The listing builds one solid part. Answer for the finished solid, in the listing's coordinates (mm). A direction names the side the tool comes from. Give positions to 0.01 mm unless a question says otherwise; leave off trailing zeros. Order: outer loops, then holes, each group sorted by start corner. A loop starts at its lowest first (then second) coordinate and runs counter-clockwise, first axis right, second up. Notation, with made-up numbers: (-9.75, 9.25) - (6.25, 9.25) arc R23 ccw to (6.25, 44.25) - close; hole circle Ø3 at (38, 17). An arc over 180 degrees is marked (long way). Write each question's results on one line, items separated by ' | '. Start each with the question number.
1. Section C-C (x = -5) is taken. Give the vertices of the cut face in (y, z), and give its area (3 significant figures).
2. Flat-ended cylindrical pins translate along their axes: pin 1 (2.5 mm diameter, centred on y = 26, z = 1.5, fed in from -X); pin 2 (1.5 mm diameter, centred on x = 1, z = 2.5, fed in from +Y); pin 3 (1.5 mm diameter, centred on y = -4.5, z = 3.5, fed in from -X). Find the tip coordinate at first contact, or state that the pin passes through.
3. Which of the six approach directions +Z, -Z, +X, -X, +Y, -Y give full straight-line access (tool end or side, diameter ignored) to faces 1 (the face through (21, 27.5, 2)), 2 (the face through (23, 7, 0))?
4. Section A-A (y = 24) is taken. Give the vertices of the cut face in (x, z), and give its area (3 significant figures).
5. Section B-B (z = 3.05) is taken. State how many separate pieces and enclosed holes the cut face has, and give its area (3 significant figures).
6. Section D-D (x = 17) is taken. Give the vertices of the cut face in (y, z), and give its area (3 significant figures).
7. Determine the mould class of faces 3 (the face through (12.86, 31.93, 2.46)), 4 (the face through (25.76, 25, 2)), 5 (the face through (44.655, 5.676, 2.465)) for opening direction X: released by +X, released by -X, zero draft, split by the parting line, or undercut.
8. Find the intervals of material crossed by L1, parallel to Y at x = 17.5, z = 4.5; L2, parallel to Y at x = 31.5, z = 4; L3, parallel to Y at x = -5, z = 2.45, in increasing order.
from build123d import *

# Parameters (mm, degrees)
SKETCH1_R           = 2
SKETCH1_W           = 10
SKETCH1_H           = 5
BOSS_EXTRUDE1_DEPTH = 5


with BuildPart() as part:
    # Sketch1 → Boss-Extrude1 (new body)
    with BuildSketch(Plane.XY):
        with BuildLine():
            Line((-1.742019887, -10.039309555), (26.411625907, -10.039309555))
            ThreePointArc((26.411625907, -10.039309555), (30.462414048, -9.182127251), (33.818749407, -6.757532642))
            Line((33.818749407, -6.757532642), (43.703561538, 4.140888457))
            ThreePointArc((43.703561538, 4.140888457), (44.664643865, 5.699695686), (44.999999787, 7.5))
            Line((44.999999787, 7.5), (44.999999787, 30.5))
            ThreePointArc((44.999999787, 30.5), (44.41421335, 31.914213562), (42.999999787, 32.5))
            Line((42.999999787, 32.5), (14.260362516, 32.5))
            ThreePointArc((14.260362516, 32.5), (12.846148953, 31.914213562), (12.260362516, 30.5))
            Line((12.260362516, 30.5), (12.260362516, 7.356217509))
            ThreePointArc((12.260362516, 7.356217509), (11.821022687, 6.295557338), (10.760362516, 5.856217509))
            Line((10.760362516, 5.856217509), (-8.340435128, 5.856217509))
            ThreePointArc((-8.340435128, 5.856217509), (-10.829871883, 3.386204984), (-11.741942625, 0))
            ThreePointArc((-11.741942625, 0), (-8.826972094, -7.096465655), (-1.742019887, -10.039309555))
        make_face()
        with Locations((-5, 0)):
            Circle(SKETCH1_R, mode=Mode.SUBTRACT)
        with Locations((20.760362516, 25)):
            Rectangle(SKETCH1_W, SKETCH1_H, mode=Mode.SUBTRACT)
        with Locations((35.760362516, 25)):
            Rectangle(SKETCH1_W, SKETCH1_H, mode=Mode.SUBTRACT)
        with Locations((20.768559845, 15.003110344)):
            Rectangle(SKETCH1_W, SKETCH1_H, mode=Mode.SUBTRACT)
        with Locations((35.768559845, 15.003110344)):
            Rectangle(SKETCH1_W, SKETCH1_H, mode=Mode.SUBTRACT)
    extrude(amount=BOSS_EXTRUDE1_DEPTH)


solid = part.part
Reported:
1) outline: (-9.49, 0) - (-2, 0) - (-2, 5) - (-9.49, 5) - close; (2, 0) - (5.86, 0) - (5.86, 5) - (2, 5) - close | area: 56.7 mm²
2) pin 1: x = 12.26 | pin 2: y = 5.86 | pin 3: x = -11.03
3) face 1: +Z, -Z | face 2: -Z, +X, -X, +Y, -Y
4) outline: (12.26, 0) - (15.76, 0) - (15.76, 5) - (12.26, 5) - close; (25.76, 0) - (30.76, 0) - (30.76, 5) - (25.76, 5) - close; (40.76, 0) - (45, 0) - (45, 5) - (40.76, 5) - close | area: 63.7 mm²
5) separate pieces: 1 | enclosed holes: 5 | area: 1,420 mm²
6) outline: (-10.04, 0) - (12.5, 0) - (12.5, 5) - (-10.04, 5) - close; (17.5, 0) - (22.5, 0) - (22.5, 5) - (17.5, 5) - close; (27.5, 0) - (32.5, 0) - (32.5, 5) - (27.5, 5) - close | area: 163 mm²
7) face 3: released by -X | face 4: undercut | face 5: released by +X
8) L1: -10.04 to 12.5, 17.5 to 22.5, 27.5 to 32.5 | L2: -8.65 to 12.5, 17.5 to 22.5, 27.5 to 32.5 | L3: -9.49 to -2, 2 to 5.86
